```python
from build123d import *

# Parameters (mm, degrees)
BOSS_EXTRUDE1_DEPTH = 29.21
BOSS_EXTRUDE2_START = -3.81
SKETCH2_R           = 3.175
BOSS_EXTRUDE2_DEPTH = 3.81
BOSS_EXTRUDE3_START = 3.81
SKETCH3_R           = 3.175
BOSS_EXTRUDE3_DEPTH = 3.81
SKETCH5_R           = 3.175
BOSS_EXTRUDE4_DEPTH = 5.2893214


with BuildPart() as part:
    # Sketch1 → Boss-Extrude1 (new body)
    with BuildSketch(Plane.XY):
        with BuildLine():
            Line((357.71784023, 212.881801123), (352.217914789, 211.608277369))
            Line((352.217914789, 211.608277369), (352.938839753, 208.494842277))
            Line((352.938839753, 208.494842277), (367.542855209, 211.876444589))
            Line((367.542855209, 211.876444589), (361.796858989, 236.691490786))
            Line((361.796858989, 236.691490786), (358.789055407, 235.995025106))
            ThreePointArc((358.789055407, 235.995025106), (361.092162023, 232.728335773), (361.482600287, 228.750507566))
            ThreePointArc((361.482600287, 228.750507566), (361.532171417, 226.454028373), (362.395514522, 224.325434315))
            ThreePointArc((362.395514522, 224.325434315), (363.554671569, 220.88901177), (362.982664296, 217.307747657))
            ThreePointArc((362.982664296, 217.307747657), (360.881852793, 214.462416261), (357.71784023, 212.881801123))
        make_face()
    extrude(amount=-BOSS_EXTRUDE1_DEPTH)

    # Sketch2 → Boss-Extrude2 (add)
    with BuildSketch(Plane(origin=(0, 0, -29.21), x_dir=(-1, 0, 0), z_dir=(0, 0, -1)).offset(BOSS_EXTRUDE2_START)):
        with BuildLine():
            Line((-347.192843533, 233.309888473), (-352.217914789, 211.608277369))
            Line((-352.217914789, 211.608277369), (-357.71784023, 212.881801123))
            ThreePointArc((-357.71784023, 212.881801123), (-363.018157919, 217.393089456), (-362.395514522, 224.325434315))
            ThreePointArc((-362.395514522, 224.325434315), (-361.532171417, 226.454028373), (-361.482600287, 228.750507566))
            ThreePointArc((-361.482600287, 228.750507566), (-361.092162023, 232.728335773), (-358.789055407, 235.995025106))
            Line((-358.789055407, 235.995025106), (-347.192843533, 233.309888473))
        make_face()
        with Locations((-356.009914651, 220.257763535)):
            Circle(SKETCH2_R, mode=Mode.SUBTRACT)
        with Locations((-353.754071424, 230)):
            Circle(SKETCH2_R, mode=Mode.SUBTRACT)
    extrude(amount=BOSS_EXTRUDE2_DEPTH)

    # Sketch3 → Boss-Extrude3 (add)
    # profile 1 of 2: a face of its own
    with BuildSketch(Plane.XY.offset(BOSS_EXTRUDE3_START)):
        with BuildLine():
            Line((358.789055407, 235.995025106), (347.192843533, 233.309888473))
            Line((347.192843533, 233.309888473), (352.217914789, 211.608277369))
            Line((352.217914789, 211.608277369), (357.71784023, 212.881801123))
            ThreePointArc((357.71784023, 212.881801123), (363.018157919, 217.393089456), (362.395514522, 224.325434315))
            ThreePointArc((362.395514522, 224.325434315), (361.532171417, 226.454028373), (361.482600287, 228.750507566))
            ThreePointArc((361.482600287, 228.750507566), (361.092162023, 232.728335773), (358.789055407, 235.995025106))
        make_face()
        with Locations(Location((356.009914651, 220.257763535, 0), (0, 0, 180))):
            Circle(SKETCH3_R, mode=Mode.SUBTRACT)
        with Locations(Location((353.754071424, 230, 0), (0, 0, 180))):
            Circle(SKETCH3_R, mode=Mode.SUBTRACT)
    # profile 2 of 2: a face of its own
    with BuildSketch(Plane.XY.offset(BOSS_EXTRUDE3_START)):
        with BuildLine():
            ThreePointArc((361.482600287, 228.750507566), (361.532171417, 226.454028373), (362.395514522, 224.325434315))
            ThreePointArc((362.395514522, 224.325434315), (363.018157919, 217.393089456), (357.71784023, 212.881801123))
            Line((357.71784023, 212.881801123), (352.217914789, 211.608277369))
            Line((352.217914789, 211.608277369), (352.938839753, 208.494842277))
            Line((352.938839753, 208.494842277), (367.542855209, 211.876444589))
            Line((367.542855209, 211.876444589), (361.796858989, 236.691490786))
            Line((361.796858989, 236.691490786), (358.789055407, 235.995025106))
            ThreePointArc((358.789055407, 235.995025106), (361.092162023, 232.728335773), (361.482600287, 228.750507566))
        make_face()
    extrude(amount=-BOSS_EXTRUDE3_DEPTH)

    # Sketch5 → Boss-Extrude4 (add)
    with BuildSketch(Plane(origin=(0, 211.876444589, 0), x_dir=(1, 0, 0), z_dir=(0, 1, 0))):
        Polygon((353.064855209, 73.907779308), (416.564855209, 73.907779308), (416.564855209, 47.589788729), (373.814351909, 47.589788729), (375.477626365, -54.010211271), (335.779852437, -53.851377651), (335.779852437, -22.612220692), (354.644965943, -22.612220692), align=None)
        with Locations(Location((404.073297936, 63.14930327, 0), (0, 0, 270))):
            Circle(SKETCH5_R, mode=Mode.SUBTRACT)
        with Locations(Location((352.49755845, -42.393532045, 0), (0, 0, 270))):
            Circle(SKETCH5_R, mode=Mode.SUBTRACT)
    extrude(amount=-BOSS_EXTRUDE4_DEPTH)


solid = part.part
```
Here's how the part is built. I have some questions about the finished solid (model axes, mm). A direction names the side the tool comes from. Coordinates: 2 decimals unless noted, no trailing zeros. Loops run counter-clockwise (first coordinate to the right, second up) from the corner with the lowest first, then second, coordinate; pieces in that order, holes last. Notation, with made-up numbers: M 3,-28.75 L 30,-28.75 A13 cw 30,-10.75 Z; hole C 75.25,69.25 d6. An arc over 180 degrees is marked long. One line per item, written item: value.
1. Imagine slicing it at A-A (y = 230). List the corners of the cut face in (x, z) for me, and give its area (3 significant figures).
Geometry says:
outline: M 347.96,-29.21 L 350.58,-29.21 L 350.58,-25.4 L 347.96,-25.4 Z; M 347.96,0 L 350.58,0 L 350.58,3.81 L 347.96,3.81 Z; M 356.93,-29.21 L 363.35,-29.21 L 363.35,3.81 L 356.93,3.81 L 356.93,0 L 361.58,0 L 361.58,-25.4 L 356.93,-25.4 Z
area: 114 mm2
2. Please list where these lines run through material, in increasing order: probe 1 along Z at (x, y) = (363, 220); probe 2 along Y at (x, z) = (340, 46); probe 3 along Z at (x, y) = (362, 214).
Geometry says:
probe 1: z = -29.21 to -25.4, 0 to 3.81
probe 2: y = 206.59 to 211.88
probe 3: z = -29.21 to 3.81
3. On a 3-axis mill with a long thin cutter (end or side, diameter ignored), from which of +Z, -Z, +X, -X, +Y, -Y can I reach the whole of each face in a straight line? I mean faces 4 (the flat face through (357, 224, 0)), 5 (the flat face through (335.78, 209, 38)). Say none if no direction works.
Geometry says:
face 4: -X
face 5: +Z, -Z, -X, +Y, -Y
4. Will these pins go through, and if not, where does the flat tip stop? pin 1 Ø8.5 at (x, y) = (356.01, 220.26) entering from +Z; pin 2 Ø10 at (x, y) = (352.5, 220) entering from -Z; pin 3 Ø3 at (x, z) = (377.5, -23) entering from -Y; pin 4 Ø4 at (x, z) = (401, -61) entering from +Y.
Geometry says:
pin 1: stops at z = 3.81
pin 2: stops at z = -29.21
pin 3: passes through
pin 4: stops at y = 211.88
5. Thinking about a two-plate mould opening in Y: for faces 1 (the flat face through (359, 223, 3.81)), 2 (the flat face through (364.71, 224.11, -12.47)), 3 (the cylindrical face through (356.926, 229.86, 1.932)), which applies, +Y half, -Y half, draft (parallel to the pull), parting line (faces both ways), or undercut?
Geometry says:
face 1: draft
face 2: +Y half
face 3: undercut
6. Imagine slicing it at C-C (x = 409.5). List the corners of the cut face in (y, z) for me, and give its area (3 significant figures).
Geometry says:
outline: M 206.59,-73.91 L 211.88,-73.91 L 211.88,-47.59 L 206.59,-47.59 Z
area: 139 mm2
7. Imagine slicing it at B-B (z = -64). List the corners of the cut face in (x, y) for me, and give its area (3 significant figures).
Geometry says:
outline: M 353.23,206.59 L 401.01,206.59 L 401.01,211.88 L 353.23,211.88 Z; M 407.13,206.59 L 416.56,206.59 L 416.56,211.88 L 407.13,211.88 Z
area: 303 mm2
8. Imagine slicing it at D-D (z = -18). List the corners of the cut face in (x, y) for me, and give its area (3 significant figures).
Geometry says:
outline: M 352.22,211.61 L 352.94,208.49 L 353.98,208.74 L 353.98,206.59 L 374.3,206.59 L 374.3,211.88 L 367.54,211.88 L 361.8,236.69 L 358.79,236 A7.83 cw 361.48,228.75 A6.35 ccw 362.4,224.33 A7.57 cw 357.72,212.88 Z
area: 190 mm2
